Part model, mm, in its own coordinate system. A direction names the side the tool comes from. Coordinates: 2 decimals unless noted, no trailing zeros. Write each loop counter-clockwise with the first axis right and the second up, starting at its lowest first coordinate (ties: lowest second). Pieces come first, ordered by that corner, then holes. Notation, with made-up numbers: (-4, -21) - (38, -21) arc R29 cw to (38, 4) - close; hole circle Ø10 at (23.25, 28). An arc over 180 degrees is marked (long way). Write each question's results on one line, items separated by ' | '.
from build123d import *

# Parameters (mm, degrees)
SKETCH1_R           = 3.2
BOSS_EXTRUDE1_DEPTH = 3.175
SKETCH3_R           = 3.2
BOSS_EXTRUDE2_DEPTH = 3.175
FILLET1_R           = 6.5
SKETCH6_R           = 1.45
CUT_EXTRUDE4_DEPTH  = 86.409103367
CUT_EXTRUDE14_DEPTH = 86.409103367
CUT_EXTRUDE13_DEPTH = 86.409103367
FILLET2_R           = 8
SKETCH9_R           = 1.25
CUT_EXTRUDE15_DEPTH = 86.409103367


with BuildPart() as part:
    # Sketch1 → Boss-Extrude1 (new body)
    with BuildSketch(Plane.XY):
        Polygon((0, 36.5), (-10, 35.30709832), (-16, 29), (-56.5, 27.5), (-76.5, 14), (-76.5, -14), (-56.5, -27.5), (-16, -29), (-10, -35.30709832), (0, -36.5), (10, -35.30709832), (16, -29), (56.5, -27.5), (76.5, -14), (76.5, 14), (56.5, 27.5), (16, 29), (10, 35.30709832), align=None)
        with Locations((0, 30)):
            Circle(SKETCH1_R, mode=Mode.SUBTRACT)
        with Locations(Location((0, -30, 0), (0, 0, 180))):
            Circle(SKETCH1_R, mode=Mode.SUBTRACT)
    extrude(amount=BOSS_EXTRUDE1_DEPTH)

    # Sketch3 → Boss-Extrude2 (add)
    # profile 1 of 4: a face of its own
    with BuildSketch(Plane.XY.offset(3.175)):
        Polygon((-56.5, 27.5), (-65, 32.5), (-80.3, 31), (-73.537037037, 16), align=None)
        with Locations((-70.5, 25.5)):
            Circle(SKETCH3_R, mode=Mode.SUBTRACT)
    # profile 2 of 4: a face of its own
    with BuildSketch(Plane.XY.offset(3.175)):
        Polygon((73.537037037, 16), (56.5, 27.5), (65, 32.5), (80.3, 31), align=None)
        with Locations(Location((70.5, 25.5, 0), (0, 0, 180))):
            Circle(SKETCH3_R, mode=Mode.SUBTRACT)
    # profile 3 of 4: a face of its own
    with BuildSketch(Plane.XY.offset(3.175)):
        Polygon((56.5, -27.5), (65, -32.5), (80.3, -31), (73.537037037, -16), align=None)
        with Locations((70.5, -25.5)):
            Circle(SKETCH3_R, mode=Mode.SUBTRACT)
    # profile 4 of 4: a face of its own
    with BuildSketch(Plane.XY.offset(3.175)):
        Polygon((-73.537037037, -16), (-56.5, -27.5), (-65, -32.5), (-80.3, -31), align=None)
        with Locations(Location((-70.5, -25.5, 0), (0, 0, 180))):
            Circle(SKETCH3_R, mode=Mode.SUBTRACT)
    extrude(amount=-BOSS_EXTRUDE2_DEPTH)

    # Fillet1
    fillet1_edges = [part.edges().sort_by_distance(p)[0] for p in [
        (-80.3, 31, 1.5875),
        (80.3, 31, 1.5875),
        (80.3, -31, 1.5875),
        (-80.3, -31, 1.5875),
    ]]
    fillet(fillet1_edges, radius=FILLET1_R)

    # Sketch6 → Cut-Extrude4 (cut, through all)
    with BuildSketch(Plane(origin=(0, 0, 0), x_dir=(-1, 0, 0), z_dir=(0, 0, -1))):
        with Locations((8, 26)):
            Circle(SKETCH6_R)
        with Locations((-8, 26)):
            Circle(SKETCH6_R)
        with Locations((-8, -26)):
            Circle(SKETCH6_R)
        with Locations((8, -26)):
            Circle(SKETCH6_R)
    extrude(amount=-CUT_EXTRUDE4_DEPTH, mode=Mode.SUBTRACT)

    # Sketch8 → Cut-Extrude14 (cut, through all)
    with BuildSketch(Plane.XY.offset(3.175)):
        Polygon((-75.690069736, 20.775346347), (-68.5, 16.819040498), (-68.5, -16.819040498), (-75.690069736, -20.775346347), (-83.497643109, -20.775346347), (-83.497643109, 20.775346347), align=None)
        Polygon((75.690069736, -20.775346347), (68.5, -16.819040498), (68.5, 16.819040498), (75.690069736, 20.775346347), (83.497643109, 20.775346347), (83.497643109, -20.775346347), align=None)
    extrude(amount=-CUT_EXTRUDE14_DEPTH, mode=Mode.SUBTRACT)

    # Sketch7 → Cut-Extrude13 (cut, through all)
    with BuildSketch(Plane.XY.offset(3.175)):
        Polygon((0, 21.290184322), (-20.449646359, 23.681667258), (-55.655570018, 22.377744159), (-64.5, 16.407753921), (-64.5, -16.407753921), (-55.655570018, -22.377744159), (-20.449646359, -23.681667258), (0, -21.290184322), (20.449646359, -23.681667258), (55.655570018, -22.377744159), (64.5, -16.407753921), (64.5, 16.407753921), (55.655570018, 22.377744159), (20.449646359, 23.681667258), align=None)
    extrude(amount=-CUT_EXTRUDE13_DEPTH, mode=Mode.SUBTRACT)

    # Fillet2
    # the kernel refuses this fillet: 8 mm, written as the material it adds along each edge
    with BuildSketch(Plane(origin=(68.5, 16.819040498, 3.175), x_dir=(0.8761249486576493, 0.48208409467605473, 0), z_dir=(0, 0, -1)), Plane(origin=(68.5, -16.819040498, 3.175), x_dir=(0, 1, 0), z_dir=(0, 0, -1))) as fillet2_piece_1:
        with BuildLine():
            CenterArc((FILLET2_R * 0.591143884348, FILLET2_R), FILLET2_R, 208.821606211, 61.178393789)
            Line((-FILLET2_R * 0.284981064309, FILLET2_R * 0.517915905324), (0, 0))
            Line((0, 0), (FILLET2_R * 0.591143884348, 0))
        make_face()
    extrude(amount=3.175)
    with BuildSketch(Plane(origin=(-68.5, -16.819040498, 3.175), x_dir=(0, 1, 0), z_dir=(0, 0, -1)), Plane(origin=(-68.5, 16.819040498, 3.175), x_dir=(-0.8761249486576493, 0.48208409467605473, 0), z_dir=(0, 0, -1))) as fillet2_piece_2:
        with BuildLine():
            CenterArc((FILLET2_R * 0.591143884348, -FILLET2_R), FILLET2_R, 90, 61.178393789)
            Line((-FILLET2_R * 0.284981064309, -FILLET2_R * 0.517915905324), (0, 0))
            Line((0, 0), (FILLET2_R * 0.591143884348, 0))
        make_face()
    extrude(amount=3.175)
    # the kernel refuses this fillet: 8 mm, written as the material it takes off along each edge
    with BuildSketch(Plane(origin=(75.690069736, 20.775346347, 9.774776334), x_dir=(0.4110197276210946, 0.911626449542948, 0), z_dir=(0, 0, -1))) as fillet2_2_piece_1:
        with BuildLine():
            CenterArc((2.693587302, -7.982087138), FILLET2_R, 93.834919038, 33.074566144)
            Line((-2.110833522, -1.585405143), (0, 0))
            Line((0, 0), (2.158531299, 0))
        make_face()
    extrude(amount=16.374552669, mode=Mode.SUBTRACT)
    with BuildSketch(Plane(origin=(75.690069736, -20.775346347, 9.774776334), x_dir=(-0.8761249486576492, 0.48208409467605506, 0), z_dir=(0, 0, -1))) as fillet2_2_piece_2:
        with BuildLine():
            CenterArc((2.639910534, -8), FILLET2_R, 90, 33.074566144)
            Line((-1.725929787, -1.29631159), (0, 0))
            Line((0, 0), (2.639910534, 0))
        make_face()
    extrude(amount=16.374552669, mode=Mode.SUBTRACT)
    with BuildSketch(Plane(origin=(-75.690069736, -20.775346347, 9.774776334), x_dir=(0.8761249486576499, 0.48208409467605357, 0), z_dir=(0, 0, -1))) as fillet2_2_piece_3:
        with BuildLine():
            CenterArc((2.639910534, 8), FILLET2_R, 236.925433856, 33.074566144)
            Line((-1.725929787, 1.29631159), (0, 0))
            Line((0, 0), (2.639910534, 0))
        make_face()
    extrude(amount=16.374552669, mode=Mode.SUBTRACT)
    with BuildSketch(Plane(origin=(-75.690069736, 20.775346347, 9.774776334), x_dir=(-0.4110197276210959, 0.9116264495429475, 0), z_dir=(0, 0, -1))) as fillet2_2_piece_4:
        with BuildLine():
            CenterArc((2.693587302, 7.982087138), FILLET2_R, 233.090514818, 33.074566144)
            Line((-2.110833522, 1.585405143), (0, 0))
            Line((0, 0), (2.158531299, 0))
        make_face()
    extrude(amount=16.374552669, mode=Mode.SUBTRACT)

    # Sketch9 → Cut-Extrude15 (cut, through all)
    with BuildSketch(Plane.XY.offset(3.175)):
        with Locations((-48.411790338, 25.054530897)):
            Circle(SKETCH9_R)
        with Locations(Location((48.411790338, 25.054530897, 0), (0, 0, 180))):
            Circle(SKETCH9_R)
        with Locations(Location((-48.411790338, -25.054530897, 0), (0, 0, 180))):
            Circle(SKETCH9_R)
        with Locations((48.411790338, -25.054530897)):
            Circle(SKETCH9_R)
    extrude(amount=-CUT_EXTRUDE15_DEPTH, mode=Mode.SUBTRACT)


solid = part.part
(1) Saw through at A-A on y = 9.5. Write the cut outline in (x, z) (3 decimals).
Return value:
outline: (-68.5, 0) - (-64.5, 0) - (-64.5, 3.175) - (-68.5, 3.175) - close; (64.5, 0) - (68.5, 0) - (68.5, 3.175) - (64.5, 3.175) - close
(2) Two-plate mould, pull along X, no slides. Class faces 4 (the flat face through (68.099, -32.196, 1.61)), 5 (the flat face through (-60.14, -19.35, 1.61)), 6 (the flat face through (-5.07, -35.895, 1.565)): released by +X, released by -X, zero draft, split by the parting line, or undercut.
Return value:
face 4: released by +X | face 5: undercut | face 6: released by -X
(3) Wall check: line 1 (X direction, y = -2, z = 0.4); line 2 (Y direction, x = 8.5, z = 1.8); line 3 (X direction, y = 29.5, z = 1.55). Give the ranges that are in metal, low to high. Write a range as from..to.
Return value:
line 1: x = -68.5..-64.5, 64.5..68.5 | line 2: y = -35.49..-27.36, -24.64..-22.28, 22.28..24.64, 27.36..35.49 | line 3: x = -75.71..-59.9, -15.52..-3.16, 3.16..15.52, 59.9..75.71
(4) Saw through at C-C on z = 2.5. Count the separate pieces of the cut face and the enclosed holes in it, then the cut area to 3 significant figures.
Return value:
separate pieces: 1 | enclosed holes: 15 | area: 2,660 mm^2
(5) Flat gauge pins, fed straight in: P1, Ø4, axis at x = -70.5, y = 25.5, coming from the -Z side; P2, Ø1, axis at y = -10, z = 0.5, coming from the -X side. Where does each tip first touch, or does it go through?
Return value:
P1: passes through | P2: stops at x = -68.5
(6) 3-axis set-ups, long thin cutter, end or side, ignore diameter. For faces 1 (the flat face through (68.5, 0, 2)), 2 (the flat face through (35.97, -28.26, 1.57)), 3 (the flat face through (-10.08, 22.47, 1.61)): which of +Z, -Z, +X, -X, +Y, -Y reach the whole face in a straight line?
Return value:
face 1: +Z, -Z, +X | face 2: +Z, -Z, -Y | face 3: +Z, -Z
(7) Saw through at B-B on x = 8. Write the cut outline in (y, z) (3 decimals).
Return value:
outline: (-35.546, 0) - (-27.45, 0) - (-27.45, 3.175) - (-35.546, 3.175) - close; (-24.55, 0) - (-22.226, 0) - (-22.226, 3.175) - (-24.55, 3.175) - close; (22.226, 0) - (24.55, 0) - (24.55, 3.175) - (22.226, 3.175) - close; (27.45, 0) - (35.546, 0) - (35.546, 3.175) - (27.45, 3.175) - close
